Geometry check sheet. Reference: the model listing, model coordinates, mm. Face numbers are marked on the shaded views. A direction names the side the tool comes from. Coordinates: 2 decimals unless noted, no trailing zeros. Loops run counter-clockwise (first coordinate to the right, second up) from the corner with the lowest first, then second, coordinate; pieces in that order, holes last.
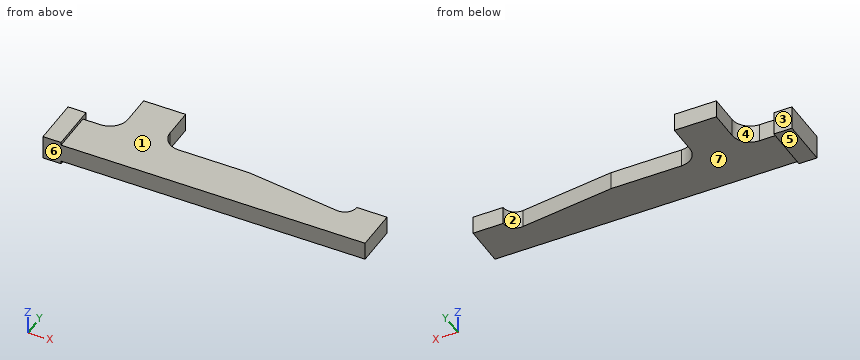
from build123d import *

# Parameters (mm, degrees)
BOSS_EXTRUDE1_DEPTH = 1.5
BOSS_EXTRUDE2_DEPTH = 2


with BuildPart() as part:
    # Sketch1 → Boss-Extrude1 (new, symmetric)
    with BuildSketch(Plane.XY):
        with BuildLine():
            Line((0, 7), (-5, 7))
            ThreePointArc((-5, 7), (-5.683439754, 5.487162066), (-7.270399626, 5))
            Line((-7.270399626, 5), (-23, 7))
            Line((-23, 7), (-34.67, 7))
            ThreePointArc((-34.67, 7), (-36.791320344, 7.878679656), (-37.67, 10))
            Line((-37.67, 10), (-37.67, 15))
            Line((-37.67, 15), (-44.67, 15))
            Line((-44.67, 15), (-44.67, 10))
            ThreePointArc((-44.67, 10), (-45.548679656, 7.878679656), (-47.67, 7))
            Line((-47.67, 7), (-50.6, 7))
            Line((-50.6, 7), (-50.6, 0))
            Line((-50.6, 0), (0, 0))
            Line((0, 0), (0, 7))
        make_face()
    extrude(amount=BOSS_EXTRUDE1_DEPTH, both=True)

    # Sketch1<6> → Boss-Extrude2 (add, symmetric)
    with BuildSketch(Plane.XY):
        Polygon((-53.6, 0), (-50.6, 0), (-50.6, 7), (-50.6, 8), (-53.6, 8), align=None)
    extrude(amount=BOSS_EXTRUDE2_DEPTH, both=True)


solid = part.part
(1) Sectioned sample at C-C on x = -2.5. Record the cut outline in (y, z).
Findings:
outline: (0, -1.5) - (7, -1.5) - (7, 1.5) - (0, 1.5) - close
(2) Scan lines: L1, parallel to X at y = 6.5, z = -1.55; L2, parallel to X at y = 7.75, z = -0.05; L3, parallel to Z at x = -16.5, y = 4.5. Record each from-to range of solid material in increasing order.
Findings:
L1: x = -53.6 to -50.6
L2: x = -53.6 to -50.6, -45.69 to -36.65
L3: z = -1.5 to 1.5
(3) Sectioned sample at A-A on y = 2.5. Record the cut outline in (x, z), and give its area (3 significant figures).
Findings:
outline: (-53.6, -2) - (-50.6, -2) - (-50.6, -1.5) - (0, -1.5) - (0, 1.5) - (-50.6, 1.5) - (-50.6, 2) - (-53.6, 2) - close
area: 164 mm2
(4) Gauge pin test, flat ends, axial feed: pin 1 Ø1 at (x, z) = (-21, 1.5) entering from +Y; pin 2 Ø1.5 at (y, z) = (13, 0.5) entering from +X; pin 3 Ø1.5 at (x, y) = (-31, 7) entering from +Z. Record the tip position at first contact, or that the pin passes through.
Findings:
pin 1: stops at y = 6.81
pin 2: stops at x = -37.67
pin 3: stops at z = 1.5
(5) Sectioned sample at D-D on y = 11. Record the cut outline in (x, z), and give its area (3 significant figures).
Findings:
outline: (-44.67, -1.5) - (-37.67, -1.5) - (-37.67, 1.5) - (-44.67, 1.5) - close
area: 21.0 mm2
(6) Draft check along X on the marked faces 1 and 2. Enter one of: +X half, -X half, draft (parallel to the pull), parting line (faces both ways), or undercut.
Findings:
face 1: draft
face 2: undercut
(7) Sectioned sample at B-B on z = -0.6. Record the cut outline in (x, y), and give its area (3 significant figures).
Findings:
outline: (-53.6, 0) - (0, 0) - (0, 7) - (-5, 7) arc R2.02 cw to (-7.27, 5) - (-23, 7) - (-34.67, 7) arc R3 cw to (-37.67, 10) - (-37.67, 15) - (-44.67, 15) - (-44.67, 10) arc R3 cw to (-47.67, 7) - (-50.6, 7) - (-50.6, 8) - (-53.6, 8) - close
area: 419 mm2
(8) Access from +Z, -Z, +X, -X, +Y, -Y to the whole of each face (thin tool, end or side, straight path). Record for the marked faces 3, 4, 5, 6 and 7.
Findings:
face 3: +Z, -Z, -X, +Y
face 4: +Z, -Z, +Y
face 5: -Z, +X, -X, +Y, -Y
face 6: +Z, -Z, +X, -X, -Y
face 7: -Z, +X, +Y, -Y
